```python
from build123d import *

# Parameters (mm, degrees)
SKETCH_2_W          = 75
SKETCH_2_H          = 40
EXTRUDE_1_DEPTH     = 2
SKETCH_3_R          = 5.05
SKETCH_3_R_2        = 1.25
CUT_EXTRUDE_1_DEPTH = 86.023526156
FILLET_1_R          = 20
SKETCH_7_W          = 2
SKETCH_7_H          = 40
EXTRUDE_3_DEPTH     = 12
SKETCH_8_R          = 1.5
CUT_EXTRUDE_2_DEPTH = 10


with BuildPart() as part:
    # 草图2 → 凸台-拉伸1 (new body)
    with BuildSketch(Plane.XY):
        with Locations((37.5, 20)):
            Rectangle(SKETCH_2_W, SKETCH_2_H)
    extrude(amount=EXTRUDE_1_DEPTH)

    # 草图3 → 切除-拉伸1 (cut, through all)
    with BuildSketch(Plane(origin=(0, 0, 0), x_dir=(-1, 0, 0), z_dir=(0, 0, -1))):
        with Locations((-26, 20)):
            Circle(SKETCH_3_R)
        with Locations((-16, 10.202041029)):
            Circle(SKETCH_3_R_2)
        with BuildLine():
            ThreePointArc((-36.446428571, 32.447274003), (-40.413244876, 12.495276677), (-21.792765741, 4.30408716))
            ThreePointArc((-21.792765741, 4.30408716), (-20.20202563, 7.059907527), (-22.957845998, 8.650647638))
            ThreePointArc((-22.957845998, 8.650647638), (-36.421884756, 14.573507751), (-33.553571429, 29.000336587))
            ThreePointArc((-33.553571429, 29.000336587), (-33.276531292, 32.170233866), (-36.446428571, 32.447274003))
        make_face()
    extrude(amount=-CUT_EXTRUDE_1_DEPTH, mode=Mode.SUBTRACT)

    # 圆角1
    fillet_1_edges = [part.edges().sort_by_distance(p)[0] for p in [
        (0, 40, 1),
        (0, 0, 1),
    ]]
    fillet(fillet_1_edges, radius=FILLET_1_R - 0.0001)  # a hair under: the kernel refuses the full size

    # 草图7 → 凸台-拉伸3 (add)
    with BuildSketch(Plane(origin=(0, 0, 0), x_dir=(-1, 0, 0), z_dir=(0, 0, -1))):
        with Locations((-74, 20)):
            Rectangle(SKETCH_7_W, SKETCH_7_H)
    extrude(amount=-EXTRUDE_3_DEPTH)

    # 草图8 → 切除-拉伸2 (cut)
    with BuildSketch(Plane.ZY.offset(-73)):
        with Locations((7, 33)):
            Circle(SKETCH_8_R)
        with Locations((7, 8)):
            Circle(SKETCH_8_R)
    extrude(amount=-CUT_EXTRUDE_2_DEPTH, mode=Mode.SUBTRACT)


solid = part.part
```
The model under review builds one solid part; all positions refer to its coordinate system, in mm. A direction names the side the tool comes from. Give positions to 0.01 mm unless a question says otherwise; leave off trailing zeros. Write each loop counter-clockwise with the first axis right and the second up, starting at its lowest first coordinate (ties: lowest second). Pieces come first, ordered by that corner, then holes.
(1) Consider section A-A, the plane z = 7. Give the boundary of the cut face in (x, y), and give its area (3 significant figures).
(2) For P1, Ø2, axis at x = 29, y = 8.5, coming from the +Z side; P2, Ø4, axis at y = 8, z = 7, coming from the -X side, all flat-tipped, find the tip position at first contact; note any pin that passes through.
(3) Consider section D-D, the plane x = 58.5. Give the boundary of the cut face in (y, z), and give its area (3 significant figures).
(4) To check wall thickness, follow L1, parallel to Y at x = 26, z = 1; L2, parallel to Y at x = 73.9, z = 7; L3, parallel to X at y = 20.5, z = 2.75. State the ranges of each line that lie inside material, in increasing order.
(5) Tool access review of faces 1 (the flat face through (36, 20, 2)), 2 (the flat face through (51, 0, 1)): name each direction out of +Z, -Z, +X, -X, +Y, -Y from which nothing blocks a thin tool from reaching the whole face with its end or side.
(6) Consider section C-C, the plane x = 16. Give the boundary of the cut face in (y, z), and give its area (3 significant figures).
(7) Consider section B-B, the plane x = 26. Give the boundary of the cut face in (y, z), and give its area (3 significant figures).
(8) The part is to be moulded in two halves that separate along X. For faces 3 (the flat face through (73, 20, 7)), 4 (the cylindrical face through (40.553, 12.77, 0.986)), 5 (the flat face through (37, 20, 0)), 6 (the flat face through (75, 20, 6)), say which applies: released by +X, released by -X, zero draft, split by the parting line, or undercut.
Returned:
1. outline: (73, 0) - (75, 0) - (75, 6.5) - (73, 6.5) - close; (73, 9.5) - (75, 9.5) - (75, 31.5) - (73, 31.5) - close; (73, 34.5) - (75, 34.5) - (75, 40) - (73, 40) - close
1. area: 68.0 mm2
2. P1: stops at z = 2
2. P2: stops at x = 73
3. outline: (0, 0) - (40, 0) - (40, 2) - (0, 2) - close
3. area: 80.0 mm2
4. L1: y = 0 to 3.75, 8.25 to 14.95, 25.05 to 40
4. L2: y = 0 to 6.5, 9.5 to 31.5, 34.5 to 40
4. L3: x = 73 to 75
5. face 1: +Z, -X, +Y, -Y
5. face 2: +Z, -Z, +X, -X, -Y
6. outline: (0.4, 0) - (8.95, 0) - (8.95, 2) - (0.4, 2) - close; (11.45, 0) - (39.6, 0) - (39.6, 2) - (11.45, 2) - close
6. area: 73.4 mm2
7. outline: (0, 0) - (3.75, 0) - (3.75, 2) - (0, 2) - close; (8.25, 0) - (14.95, 0) - (14.95, 2) - (8.25, 2) - close; (25.05, 0) - (40, 0) - (40, 2) - (25.05, 2) - close
7. area: 50.8 mm2
8. face 3: released by -X
8. face 4: undercut
8. face 5: zero draft
8. face 6: released by +X
